from build123d import *

# Parameters (mm, degrees)
SKETCH1_R           = 12.5
BOSS_EXTRUDE1_DEPTH = 17
SKETCH2_R           = 10.1
CUT_EXTRUDE1_DEPTH  = 10
SKETCH3_R           = 1.3
CUT_EXTRUDE2_DEPTH  = 10
CUT_EXTRUDE3_START  = -5
SKETCH4_R           = 12.5
SKETCH4_R_2         = 10.85
CUT_EXTRUDE3_DEPTH  = 5
BOSS_EXTRUDE2_START = -3.5
SKETCH7_R           = 11.25
SKETCH7_R_2         = 10.85
BOSS_EXTRUDE2_DEPTH = 3.5
CHAMFER1_SIZE       = 0.2


with BuildPart() as part:
    # Sketch1 → Boss-Extrude1 (new body)
    with BuildSketch(Plane(origin=(0, 0, 0), x_dir=(1, 0, 0), z_dir=(0, 1, 0))):
        with Locations(Location((0, 0, 0), (0, 0, 270))):
            Circle(SKETCH1_R)
    extrude(amount=BOSS_EXTRUDE1_DEPTH)

    # Sketch2 → Cut-Extrude1 (cut)
    with BuildSketch(Plane(origin=(0, 17, 0), x_dir=(1, 0, 0), z_dir=(0, 1, 0))):
        with Locations(Location((0, 0, 0), (0, 0, 270))):
            Circle(SKETCH2_R)
    extrude(amount=-CUT_EXTRUDE1_DEPTH, mode=Mode.SUBTRACT)

    # Sketch3 → Cut-Extrude2 (cut)
    with BuildSketch(Plane(origin=(0, 7, 0), x_dir=(1, 0, 0), z_dir=(0, 1, 0))):
        with Locations(Location((7.5, 0, 0), (0, 0, 270))):
            Circle(SKETCH3_R)
        with Locations(Location((-7.5, 0, 0), (0, 0, 270))):
            Circle(SKETCH3_R)
    extrude(amount=-CUT_EXTRUDE2_DEPTH, mode=Mode.SUBTRACT)

    # Sketch4 → Cut-Extrude3 (cut)
    with BuildSketch(Plane(origin=(0, 17, 0), x_dir=(1, 0, 0), z_dir=(0, 1, 0)).offset(CUT_EXTRUDE3_START)):
        with Locations(Location((0, 0, 0), (0, 0, 270))):
            Circle(SKETCH4_R)
        with Locations(Location((0, 0, 0), (0, 0, 270))):
            Circle(SKETCH4_R_2, mode=Mode.SUBTRACT)
    extrude(amount=CUT_EXTRUDE3_DEPTH, mode=Mode.SUBTRACT)

    # Sketch7 → Boss-Extrude2 (add)
    with BuildSketch(Plane(origin=(0, 17, 0), x_dir=(1, 0, 0), z_dir=(0, 1, 0)).offset(BOSS_EXTRUDE2_START)):
        with Locations(Location((0, 0, 0), (0, 0, 270))):
            Circle(SKETCH7_R)
        with Locations(Location((0, 0, 0), (0, 0, 270))):
            Circle(SKETCH7_R_2, mode=Mode.SUBTRACT)
    extrude(amount=BOSS_EXTRUDE2_DEPTH)

    # Chamfer1
    chamfer1_edges = [part.edges().sort_by_distance(p)[0] for p in [
        (7.5, 0, -1.3),
        (7.5, 7, -1.3),
        (-7.5, 0, -1.3),
        (-7.5, 7, -1.3),
        (0, 0, -12.5),
        (0, 17, -11.25),
    ]]
    chamfer(chamfer1_edges, length=CHAMFER1_SIZE)


solid = part.part
Work out the finished part from the listing and answer in its coordinate system (mm). A direction names the side the tool comes from. Round coordinates to 2 decimals unless told otherwise and drop trailing zeros. Order: outer loops, then holes, each group sorted by start corner. A loop starts at its lowest first (then second) coordinate and runs counter-clockwise, first axis right, second up. Notation, with made-up numbers: M -35,84 L 10,84 A13 cw 10,92 Z; hole C -36,53 d7. An arc over 180 degrees is marked long. One line per item, written item: value.
Q1. Find section A-A on x = 0. Write down the section's boundary in (y, z).
Derived:
outline: M 0,-12.3 L 0.2,-12.5 L 12,-12.5 L 12,-10.85 L 13.5,-10.85 L 13.5,-11.25 L 16.8,-11.25 L 17,-11.05 L 17,-10.1 L 7,-10.1 L 7,10.1 L 17,10.1 L 17,11.05 L 16.8,11.25 L 13.5,11.25 L 13.5,10.85 L 12,10.85 L 12,12.5 L 0.2,12.5 L 0,12.3 Z
Q2. Flat-ended cylindrical pins translate along their axes: pin 1 (6 mm diameter, centred on y = 10.5, z = -7, fed in from -X); pin 2 (6 mm diameter, centred on x = -8, z = -8.5, fed in from +Y); pin 3 (1.6 mm diameter, centred on x = -7.5, z = 0, fed in from -Y); pin 4 (1 mm diameter, centred on x = -3, y = 11.5, fed in from -Z). Find the tip coordinate at first contact, or state that the pin passes through.
Derived:
pin 1: x = -11.84
pin 2: y = 17
pin 3: through
pin 4: z = -12.25
Q3. Determine the mould class of faces 4 (the face through (-9, 17, 5)), 5 (the face through (-6.146, 12.07, -8.015)), 6 (the face through (3.26, 12.74, 10.35)), 7 (the face through (0, 0, 0)) for opening direction Y: released by +Y, released by -Y, zero draft, split by the parting line, or undercut.
Derived:
face 4: released by +Y
face 5: zero draft
face 6: undercut
face 7: released by -Y
Q4. Find section C-C on y = 7.5. Write down the section's boundary in (x, z).
Derived:
outline: C 0,0 d25; hole C 0,0 d20.2
Q5. Straight lines are drawn through the part: line 1 (X direction, y = 2.75, z = 0); line 2 (Y direction, x = -1.5, z = 5); line 3 (X direction, y = 16.25, z = -4.75). For each, find the intervals that lie inside material, in ascending order.
Derived:
line 1: -12.5 to -8.8, -6.2 to 6.2, 8.8 to 12.5
line 2: 0 to 7
line 3: -10.2 to -8.91, 8.91 to 10.2
Q6. For faces 1 (the face through (3.755, 6.017, 11.923)), 2 (the face through (1, 13.5, -11)), 3 (the face through (0, 7, 0)), determine the directions among +Z, -Z, +X, -X, +Y, -Y from which every point of the face is accessible in a straight line to the end or side of a thin tool.
Derived:
face 1: +Y, -Y
face 2: none
face 3: +Y
Q7. Find section B-B on z = 0. Give the number of separate pieces and of enclosed holes in the cut face, then the cut area to 3 significant figures.
Derived:
separate pieces: 3
enclosed holes: 0
area: 173 mm²
